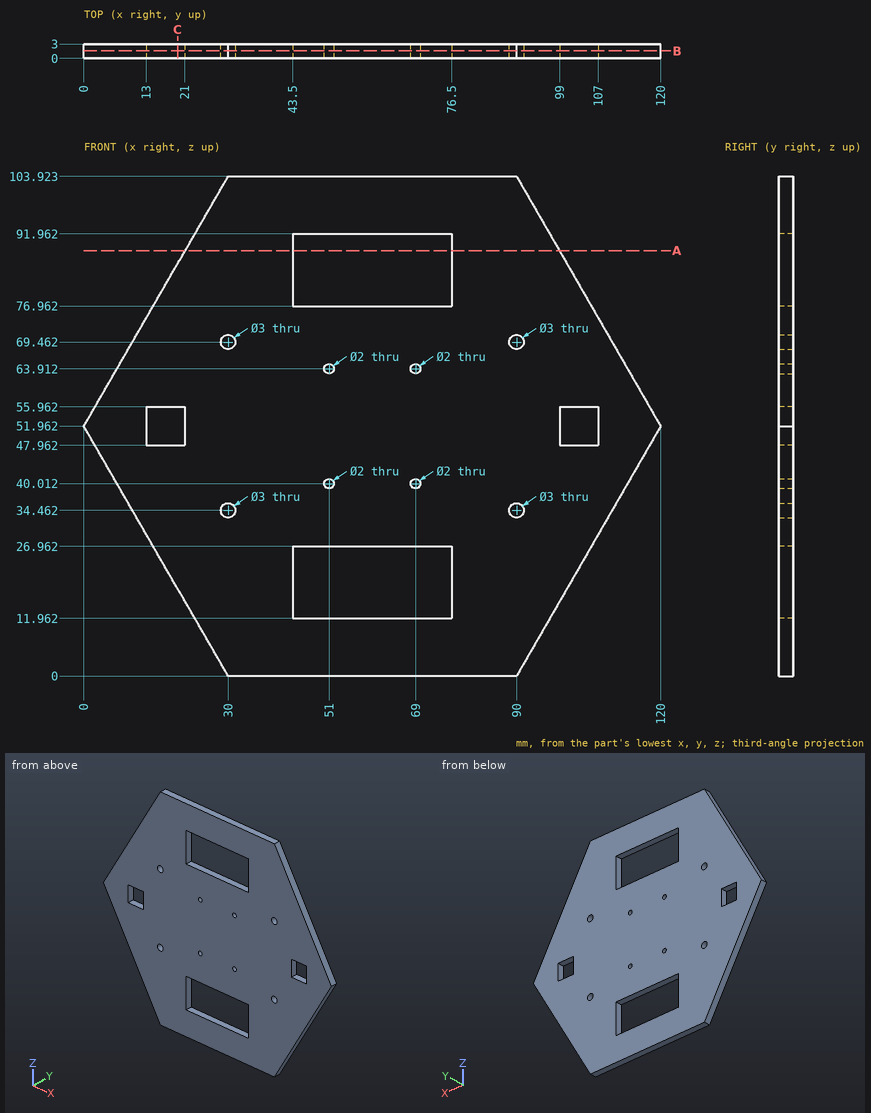
Geometry: see drawing. Coordinates: mm, zero at the bounding-box minimum. Coordinates: 2 decimals unless noted, no trailing zeros. Loops run counter-clockwise (first coordinate to the right, second up) from the corner with the lowest first, then second, coordinate; pieces in that order, holes last. Notation, with made-up numbers: M -23.75,-33.5 L 8.25,-33.5 A38 ccw 8.25,4.5 Z; hole C 79,80 d6. An arc over 180 degrees is marked long. Answer in a Markdown table with one row per item.
1. Section C-C, the plane x = 19.5. Output: boundary loops of the cut face in (y, z).
Response:
| item | result |
|---|---|
| outline | M 0,18.19 L 3,18.19 L 3,47.96 L 0,47.96 Z; M 0,55.96 L 3,55.96 L 3,85.74 L 0,85.74 Z |
2. Section A-A, the plane z = 88.5. Output: boundary loops of the cut face in (x, y) (1 decimal).
Response:
| item | result |
|---|---|
| outline | M 21.1,0 L 43.5,0 L 43.5,3 L 21.1,3 Z; M 76.5,0 L 98.9,0 L 98.9,3 L 76.5,3 Z |
3. Section B-B, the plane y = 1.55. Count the separate pieces of the cut face and the enclosed holes in it, then the cut area to 3 significant figures.
Response:
| item | result |
|---|---|
| separate pieces | 1 |
| enclosed holes | 12 |
| area | 8,190 mm2 |
4. First-contact query: pin 1 (1.5 mm diameter, centred on y = 2, z = 22, fed in from -X) (1 decimal); pin 2 (1.5 mm diameter, centred on x = 104, y = 2, fed in from +Z) (1 decimal); pin 3 (8 mm diameter, centred on x = 60.5, z = 82, fed in from +Y); pin 4 (1 mm diameter, centred on y = 1.5, z = 15.5, fed in from +X). Flat tips, straight axial feed; report the tip coordinate or a pass-through.
Response:
| item | result |
|---|---|
| pin 1 | stops at x = 16.9 |
| pin 2 | stops at z = 81 |
| pin 3 | passes through |
| pin 4 | stops at x = 99.24 |
5. Material intervals for line 1 (Z direction, x = 59.5, y = 1.6); line 2 (Z direction, x = 51, y = 1.45); line 3 (Z direction, x = 90, y = 2.2) (1 decimal), sorted ascending.
Response:
| item | result |
|---|---|
| line 1 | z = 0 to 11.96, 26.96 to 76.96, 91.96 to 103.92 |
| line 2 | z = 0 to 11.96, 26.96 to 39.01, 41.01 to 62.91, 64.91 to 76.96, 91.96 to 103.92 |
| line 3 | z = 0 to 33, 36 to 68, 71 to 103.9 |
